Autodesk Inventor part; units mm, degrees
ref_plane "YZ Plane" through (0, 0, 0) normal (1, 0, 0) x (0, 1, 0)
ref_plane "XZ Plane" through (0, 0, 0) normal (0, 1, 0) x (-1, 0, 0)
ref_plane "XY Plane" through (0, 0, 0) normal (0, 0, 1) x (1, 0, 0)
sketch "Sketch1" plane through (0, 0, 0) normal (0, 1, 0) x (-1, 0, 0)
  line L0 (10, 10) -> (-90, 10)
  line L1 (-90, 10) -> (-90, -10)
  line L2 (-90, -10) -> (10, -10)
  line L3 (10, -10) -> (10, 10)
  line L4 (-6, -15) -> (-74, -15)
  line L5 (-74, -15) -> (-74, 0)
  line L6 (-74, 0) -> (-6, 0)
  line L7 (-6, 0) -> (-6, -15)
  point P0 (0, 0)
  point P1 (-74, -10)
  point P2 (-6, -10)
  dimension "d0" = 20
  dimension "d1" = 100
  dimension "d4" = 10
  dimension "d5" = 16
  dimension "d6" = 16
extrude "Extrusion1" add sketch "Sketch1" along normal blind 950 contours L3 L2 L7 L6 L5 L1 L0
properties part number "L_PlNKA800" material "Aluminum 6061"
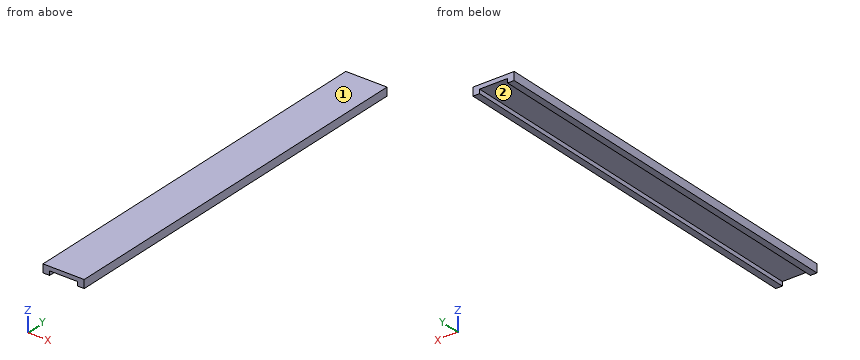
Can you work these out from the model? Positions are in its coordinate system, mm. Face numbers are marked on the shaded views. Round coordinates to 2 decimals unless told otherwise and drop trailing zeros. Loops run counter-clockwise (first coordinate to the right, second up) from the corner with the lowest first, then second, coordinate; pieces in that order, holes last. Notation, with made-up numbers: M -13,-33.5 L 42,-33.5 A29 ccw 42,-2.5 Z; hole C 76,-4.5 d11. An arc over 180 degrees is marked long. Write item = value, one per line. Start each with the question number.
(1) Suppose I cut it at C-C on x = 61. Write out the boundary of the cut face in (y, z).
(2) I need wall thicknesses on line 1 along X through (y, z) = (447.5, -5.75); line 2 along Z through (x, y) = (44, 487). Which ranges of each line are inside material? Lowest first, please.
(3) I'm going to push flat-ended pins straight in: P1, Ø5, axis at x = 27.5, z = -4, coming from the +Y side; P2, Ø6, axis at x = 50.5, y = 556.5, coming from the -Z side. Where does each tip first touch, or does it pass through?
(4) Suppose I cut it at A-A on z = -6.5. Write out the boundary of the cut face in (x, y).
(5) If we mould it in two halves opening along X, with no side actions, what happens to the marked faces 1 and 2? For each: released by +X, released by -X, zero draft, split by the parting line, or undercut.
(6) Suppose I cut it at B-B on y = 94.5. Write out the boundary of the cut face in (x, z).
Answer block:
q1.outline = M 0,0 L 950,0 L 950,10 L 0,10 Z
q2.line_1 = -10 to 6, 74 to 90
q2.line_2 = 0 to 10
q3.P1 = through
q3.P2 = 0
q4.outline = M -10,0 L 6,0 L 6,950 L -10,950 Z; M 74,0 L 90,0 L 90,950 L 74,950 Z
q5.face_1 = zero draft
q5.face_2 = undercut
q6.outline = M -10,-10 L 6,-10 L 6,0 L 74,0 L 74,-10 L 90,-10 L 90,10 L -10,10 Z
